Input: part model. Units: mm. Frame: model coordinates. Face numbers are marked on the shaded views. A direction names the side the tool comes from. Coordinates: 2 decimals unless noted, no trailing zeros. Order: outer loops, then holes, each group sorted by start corner. A loop starts at its lowest first (then second) coordinate and runs counter-clockwise, first axis right, second up. Notation, with made-up numbers: (-24, 42.25) -> (3, 42.25) arc R14 cw to (3, 63.25) -> close; hole circle Ø2 at (28.5, -1). An arc over 180 degrees is marked (long way). Use one line per item in the form item = value. Start each with the question number.
1) Pin query (flat end, axial travel): pin 1 (4 mm diameter, centred on y = 82, z = 41, fed in from -X); pin 2 (1.5 mm diameter, centred on x = 237, z = 76, fed in from +Y). Return the tip coordinate at first contact, or that it passes through.
2) Section query C-C on z = 22. Count the separate pieces of the cut face and the enclosed holes in it, then the cut area to 4 significant figures.
3) Draft query along Z for the marked faces 1, 2, 3 and 4. Return one class per face: pulls with the +Z half, pulls with the -Z half, needs draft (parallel to the pull), parting line crosses it, or undercut.
4) Section query D-D on z = 81.5. Output: boundary loops of the cut face in (x, y).
5) Section query B-B on x = 255. Output: boundary loops of the cut face in (y, z), then the cut area to 3 significant figures.
6) Access query for the marked faces 5 and 6. Directions: +Z, -Z, +X, -X, +Y, -Y. A direction counts if a zero-diameter tool reaches every point of the face in a straight line with its end or side. Return the directions, or none.
7) Ray query, line 1 along Z through (x, y) = (164, 49); line 2 along Z through (x, y) = (191, 6); line 3 along Y through (x, z) = (181, 54). Return the intervals inside material, ascending.
8) Section query A-A on y = 40.5. Output: boundary loops of the cut face in (x, z).
Autodesk Inventor part; units mm, degrees
ref_plane "YZ Plane" through (0, 0, 0) normal (1, 0, 0) x (0, 1, 0)
ref_plane "XZ Plane" through (0, 0, 0) normal (0, 1, 0) x (-1, 0, 0)
ref_plane "XY Plane" through (0, 0, 0) normal (0, 0, 1) x (1, 0, 0)
sketch "Sketch1" plane through (0, 0, 0) normal (0, 0, 1) x (1, 0, 0)
  line L0 (0, 0) -> (275, 0)
  line L1 (275, 0) -> (275, 200)
  line L2 (275, 200) -> (0, 200)
  line L3 (0, 200) -> (0, 0)
  dimension "d0" = 275
  dimension "d1" = 200
extrude "Extrusion1" add sketch "Sketch1" along normal blind 20
sketch "Sketch3" plane through (0, 0, 20) normal (0, 0, 1) x (1, 0, 0)
  line L0 (275, 0) -> (275, 200)
  line L1 (0, 200) -> (275, 200)
  line L2 (275, 200) -> (275, 0)
  line L3 (275, 0) -> (0, 0)
  line L4 (0, 0) -> (0, 200)
  point P0 (0, 0)
extrude "Extrusion3" add sketch "Sketch3" along normal blind 80
sketch "Sketch4" plane through (0, 0, 0) normal (0, -1, 0) x (1, 0, 0)
  circle A0 centre (47.5, 50) radius 17.5
  circle A1 centre (227.5, 50) radius 17.5
  line L0 (47.5, 50) -> (227.5, 50) construction
  line L1 (0, 0) -> (0, 100)
  line L2 (0, 100) -> (275, 100)
  point P0 (0, 50)
  point P1 (137.5, 50)
  point P2 (137.5, 100)
  dimension "d10" = 35
  dimension "d11" = 35
  dimension "d12" = 180
extrude "Extrusion4" cut sketch "Sketch4" against normal blind 100 contours A0
sketch "Sketch5" plane through (0, 200, 0) normal (0, 1, 0) x (1, 0, 0)
  line L0 (275, 0) -> (0, 0)
  line L1 (0, 0) -> (0, -100)
  line L2 (275, -100) -> (0, -100)
  line L3 (275, 0) -> (275, -100)
  line L4 (265, -90) -> (10, -90)
  line L5 (10, -90) -> (10, -10)
  line L6 (10, -10) -> (265, -10)
  line L7 (265, -10) -> (265, -90)
  point P0 (0, 0)
  dimension "d15" = 10
extrude "Extrusion5" cut sketch "Sketch5" against normal blind 190 contours L4 L5 L6 L7
sketch "Sketch6" plane through (0, 0, 0) normal (-1, 0, 0) x (0, 0, 1)
  line L0 (0, 200) -> (100, 200)
  line L1 (0, 200) -> (0, 0)
  line L2 (100, 200) -> (0, 200)
  line L3 (0, 200) -> (0, 190)
  line L4 (0, 190) -> (100, 190)
  line L5 (100, 190) -> (100, 200)
  dimension "d18" = 10
extrude "Extrusion6" cut sketch "Sketch6" against normal through all
sketch "Sketch7" plane through (0, 190, 100) normal (0, 1, 0) x (1, 0, 0)
  line L0 (275, 100) -> (275, 0) construction
  line L1 (0, 100) -> (275, 100) construction
  line L2 (0, 0) -> (0, 100) construction
  line L3 (275, 0) -> (0, 0) construction
  line L4 (265, 10) -> (265, 90) construction
  line L5 (10, 10) -> (265, 10) construction
  line L6 (10, 90) -> (10, 10) construction
  line L7 (265, 90) -> (10, 90) construction
  line L8 (270, 5) -> (270, 95) construction
  line L9 (270, 95) -> (5, 95) construction
  line L10 (5, 95) -> (5, 5) construction
  line L11 (5, 5) -> (270, 5) construction
  circle A0 centre (270, 5) radius 2.5
  circle A1 centre (270, 95) radius 2.5
  circle A2 centre (5, 95) radius 2.5
  circle A3 centre (5, 5) radius 2.5
  point P0 (0, 100)
  dimension "d21" = 5
  dimension "d22" = 5
  dimension "d23" = 5
  dimension "d24" = 5
  dimension "d25" = 5
extrude "Extrusion7" cut sketch "Sketch7" against normal blind 25
sketch "Sketch8" plane through (0, 0, 0) normal (0, -1, 0) x (1, 0, 0)
  line L0 (82, 15) -> (85, 15)
  line L1 (85, 15) -> (85, 35)
  line L2 (85, 35) -> (82, 35)
  line L3 (82, 35) -> (82, 15)
  line L4 (0, 0) -> (0, 100)
  line L5 (0, 0) -> (275, 0)
  line L6 (97, 15) -> (97, 35)
  line L7 (97, 35) -> (94, 35)
  line L8 (94, 35) -> (94, 15)
  line L9 (94, 15) -> (97, 15)
  line L10 (109, 15) -> (109, 35)
  line L11 (109, 35) -> (106, 35)
  line L12 (106, 35) -> (106, 15)
  line L13 (106, 15) -> (109, 15)
  line L14 (121, 15) -> (121, 35)
  line L15 (121, 35) -> (118, 35)
  line L16 (118, 35) -> (118, 15)
  line L17 (118, 15) -> (121, 15)
  line L18 (133, 15) -> (133, 35)
  line L19 (133, 35) -> (130, 35)
  line L20 (130, 35) -> (130, 15)
  line L21 (130, 15) -> (133, 15)
  line L22 (145, 15) -> (145, 35)
  line L23 (145, 35) -> (142, 35)
  line L24 (142, 35) -> (142, 15)
  line L25 (142, 15) -> (145, 15)
  line L26 (157, 15) -> (157, 35)
  line L27 (157, 35) -> (154, 35)
  line L28 (154, 35) -> (154, 15)
  line L29 (154, 15) -> (157, 15)
  line L30 (169, 15) -> (169, 35)
  line L31 (169, 35) -> (166, 35)
  line L32 (166, 35) -> (166, 15)
  line L33 (166, 15) -> (169, 15)
  line L34 (181, 15) -> (181, 35)
  line L35 (181, 35) -> (178, 35)
  line L36 (178, 35) -> (178, 15)
  line L37 (178, 15) -> (181, 15)
  line L38 (193, 15) -> (193, 35)
  line L39 (193, 35) -> (190, 35)
  line L40 (190, 35) -> (190, 15)
  line L41 (190, 15) -> (193, 15)
  line L42 (205, 15) -> (205, 35)
  line L43 (205, 35) -> (202, 35)
  line L44 (202, 35) -> (202, 15)
  line L45 (202, 15) -> (205, 15)
  line L46 (217, 15) -> (217, 35)
  line L47 (217, 35) -> (214, 35)
  line L48 (214, 35) -> (214, 15)
  line L49 (214, 15) -> (217, 15)
  line L50 (229, 15) -> (229, 35)
  line L51 (229, 35) -> (226, 35)
  line L52 (226, 35) -> (226, 15)
  line L53 (226, 15) -> (229, 15)
  line L54 (241, 15) -> (241, 35)
  line L55 (241, 35) -> (238, 35)
  line L56 (238, 35) -> (238, 15)
  line L57 (238, 15) -> (241, 15)
  dimension "d28" = 3
  dimension "d29" = 20
  dimension "d30" = 82
  dimension "d31" = 15
  dimension "d34" = 12
extrude "Extrusion8" cut sketch "Sketch8" against normal through all
sketch "Sketch2" plane through (275, 0, 100) normal (1, 0, 0) x (0, 0, -1)
  circle A0 centre (70, 125) radius 3
  line L0 (100, 0) -> (0, 0)
  line L1 (100, 0) -> (100, 190)
  dimension "d4" = 6
  dimension "d45" = 125
  dimension "d46" = 30
extrude "Extrusion2" cut sketch "Sketch2" against normal through all
sketch "Sketch10" plane through (0, 190, 100) normal (0, 1, 0) x (1, 0, 0)
  line L0 (0, 100) -> (275, 100)
  line L1 (275, 0) -> (0, 0)
  line L2 (0, 100) -> (137.5, 100)
  line L3 (137.5, 100) -> (137.5, 0)
  line L4 (137.5, 0) -> (0, 0)
  line L5 (0, 0) -> (0, 100)
extrude "Extrusion10" cut sketch "Sketch10" against normal through all
sketch "Sketch12" plane through (0, 0, 100) normal (0, 0, 1) x (1, 0, 0)
  line L0 (275, 0) -> (275, 190)
  line L1 (137.5, 190) -> (137.5, 0)
  line L2 (275, 190) -> (137.5, 190)
  line L3 (137.5, 190) -> (137.5, 95)
  line L4 (137.5, 95) -> (275, 95)
  line L5 (275, 95) -> (275, 190)
  point P0 (0, 0)
  dimension "d49" = 95
extrude "Extrusion11" cut sketch "Sketch12" against normal through all
properties part number "HA005" material "ABS Plastic"
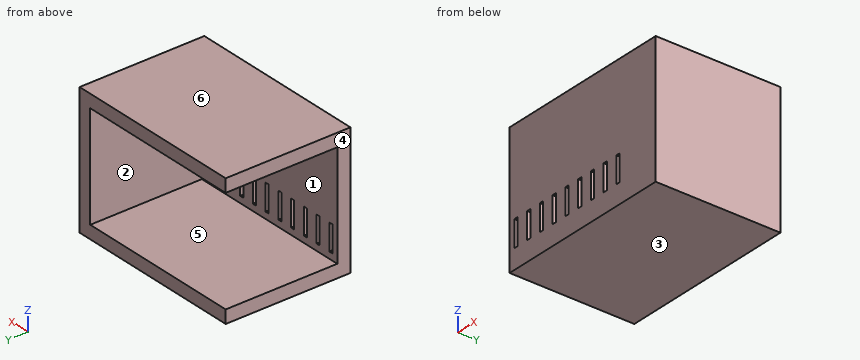
Answers below:
q1.pin_1 = 265
q1.pin_2 = 10
q2.separate_pieces = 10
q2.enclosed_holes = 0
q2.area = 1,955 mm^2
q3.face_1 = undercut
q3.face_2 = undercut
q3.face_3 = pulls with the -Z half
q3.face_4 = needs draft
q4.outline = (137.5, 0) -> (275, 0) -> (275, 95) -> (265, 95) -> (265, 10) -> (137.5, 10) -> close
q5.outline = (0, 0) -> (95, 0) -> (95, 10) -> (10, 10) -> (10, 90) -> (95, 90) -> (95, 100) -> (0, 100) -> close
q5.area = 2,700 mm^2
q6.face_5 = -X, +Y
q6.face_6 = +Z, +X, -X, +Y, -Y
q7.line_1 = 0 to 10, 90 to 100
q7.line_2 = 0 to 15, 35 to 100
q7.line_3 = 0 to 10
q8.outline = (137.5, 0) -> (275, 0) -> (275, 100) -> (137.5, 100) -> (137.5, 90) -> (265, 90) -> (265, 10) -> (137.5, 10) -> close
